Could you check a few things on this model? Use its own coordinates, in mm. A direction names the side the tool comes from. Give positions to 0.01 mm unless a question says otherwise; leave off trailing zeros. Order: outer loops, then holes, each group sorted by start corner. A loop starts at its lowest first (then second) coordinate and runs counter-clockwise, first axis right, second up. Notation, with made-up numbers: (47, 38.5) - (69, 38.5) arc R16 cw to (69, 47.5) - close; hole circle Ø7 at (-12, 69.25). An arc over 180 degrees is marked (long way). Put each result on its own line as item: value.
from build123d import *

# Parameters (mm, degrees)
SKETCH1_W           = 38
SKETCH1_H           = 38
BOSS_EXTRUDE1_DEPTH = 1.5
SKETCH2_R           = 17.5
BOSS_EXTRUDE2_DEPTH = 10
SKETCH3_R           = 14
BOSS_EXTRUDE3_DEPTH = 40.5
SKETCH4_R           = 12.5
CUT_EXTRUDE1_DEPTH  = 3
SKETCH5_R           = 1.478595514
BOSS_EXTRUDE4_DEPTH = 20
SKETCH6_W           = 22
SKETCH6_H           = 1.5
BOSS_EXTRUDE5_DEPTH = 20


with BuildPart() as part:
    # Sketch1 → Boss-Extrude1 (new body)
    with BuildSketch(Plane(origin=(0, 0, 0), x_dir=(1, 0, 0), z_dir=(0, 1, 0))):
        with Locations((-5.358974359, 7.185897436)):
            Rectangle(SKETCH1_W, SKETCH1_H)
    extrude(amount=BOSS_EXTRUDE1_DEPTH)

    # Sketch2 → Boss-Extrude2 (add)
    with BuildSketch(Plane(origin=(0, 1.5, 0), x_dir=(1, 0, 0), z_dir=(0, 1, 0))):
        with Locations((-5.358974359, 7.185897436)):
            Circle(SKETCH2_R)
    extrude(amount=BOSS_EXTRUDE2_DEPTH)

    # Sketch3 → Boss-Extrude3 (add)
    with BuildSketch(Plane(origin=(0, 11.5, 0), x_dir=(1, 0, 0), z_dir=(0, 1, 0))):
        with Locations((-5.358974359, 7.185897436)):
            Circle(SKETCH3_R)
    extrude(amount=BOSS_EXTRUDE3_DEPTH)

    # Sketch4 → Cut-Extrude1 (cut)
    with BuildSketch(Plane(origin=(0, 52, 0), x_dir=(1, 0, 0), z_dir=(0, 1, 0))):
        with Locations((-5.358974359, 7.185897436)):
            Circle(SKETCH4_R)
    extrude(amount=-CUT_EXTRUDE1_DEPTH, mode=Mode.SUBTRACT)

    # Sketch5 → Boss-Extrude4 (add)
    with BuildSketch(Plane(origin=(0, 0, 0), x_dir=(0, 0, -1), z_dir=(1, 0, 0))):
        with Locations((6.558582487, 32.23)):
            Circle(SKETCH5_R)
    extrude(amount=BOSS_EXTRUDE4_DEPTH)

    # Sketch6 → Boss-Extrude5 (add)
    with BuildSketch(Plane.XY.offset(11.814102564)):
        with Locations((-5.358974359, 0.75)):
            Rectangle(SKETCH6_W, SKETCH6_H)
    extrude(amount=BOSS_EXTRUDE5_DEPTH)


solid = part.part
1) Suppose I cut it at D-D, the plane x = -13. List the corners of the cut face in (y, z) for me.
Filled in:
outline: (0, -26.19) - (1.5, -26.19) - (1.5, -22.93) - (11.5, -22.93) - (11.5, -18.92) - (52, -18.92) - (52, -17.08) - (49, -17.08) - (49, 2.71) - (52, 2.71) - (52, 4.55) - (11.5, 4.55) - (11.5, 8.56) - (1.5, 8.56) - (1.5, 31.81) - (0, 31.81) - close
2) We'd pull the mould along Y, two halves only. Please class faces 4 (the cylindrical face through (14.159, 30.787, -6.238)), 5 (the flat face through (-6, 1, -26.186)), 6 (the flat face through (-6, 49, -7)): pulls with the +Y half, pulls with the -Y half, needs draft (parallel to the pull), parting line crosses it, or undercut.
Filled in:
face 4: undercut
face 5: needs draft
face 6: pulls with the +Y half
3) Suppose I cut it at A-A, the plane x = -3.5. List the corners of the cut face in (y, z) for me, and give its area (3 significant figures).
Filled in:
outline: (0, -26.19) - (1.5, -26.19) - (1.5, -24.59) - (11.5, -24.59) - (11.5, -21.06) - (52, -21.06) - (52, -19.55) - (49, -19.55) - (49, 5.18) - (52, 5.18) - (52, 6.69) - (11.5, 6.69) - (11.5, 10.22) - (1.5, 10.22) - (1.5, 31.81) - (0, 31.81) - close
area: 1,480 mm^2
4) Suppose I cut it at B-B, the plane z = 14. List the corners of the cut face in (x, y) for me.
Filled in:
outline: (-16.36, 0) - (5.64, 0) - (5.64, 1.5) - (-16.36, 1.5) - close
5) I'm going to push flat-ended pins straight in: pin 1 (3 mm diameter, centred on y = 37.5, z = 2.5, fed in from +X); pin 2 (4 mm diameter, centred on x = -6, y = 13, fed in from +Z); pin 3 (1.6 mm diameter, centred on x = 10, y = 0.5, fed in from +Z). Where does each tip first touch, or does it pass through?
Filled in:
pin 1: stops at x = 6
pin 2: stops at z = 10.31
pin 3: stops at z = 11.81
6) If I drill on line 1 (Y direction, x = -17.5, z = -20.5); line 2 (Y direction, x = -3, z = 8.5); line 3 (X direction, y = 49.5, z = -6), over which ranges is the centre line in solid material (lowest first)? Write a range as [from, to].
Filled in:
line 1: y = [0, 1.5]
line 2: y = [0, 11.5]
line 3: x = [-19.31, -17.8], [7.08, 8.59]
7) Suppose I cut it at C-C, the plane y = 32.23. List the corners of the cut face in (x, z) for me.
Filled in:
outline: (8.48, -5.08) arc R14 ccw (long way) to (8.62, -8.04) - (20, -8.04) - (20, -5.08) - close
8) Which directions (+Z, -Z, +X, -X, +Y, -Y) give clear straight access to the entire face, cutting with the end or side of a thin tool? Please do faces 1 (the flat face through (5.641, 1, 22)), 2 (the cylindrical face through (0.409, 50.521, 3.904)), 3 (the flat face through (-20, 1, 11.814)).
Filled in:
face 1: +Z, +X, +Y, -Y
face 2: +Y
face 3: +Z, -X, +Y, -Y
